Check sheet for the modelled part. Datum: model origin and axes. Units: mm. A direction names the side the tool comes from. Round coordinates to 2 decimals unless told otherwise and drop trailing zeros. Order: outer loops, then holes, each group sorted by start corner. A loop starts at its lowest first (then second) coordinate and runs counter-clockwise, first axis right, second up. Notation, with made-up numbers: M 26.25,49 L 55.25,49 A29 ccw 55.25,74 Z; hole C -34,42 d8. An arc over 180 degrees is marked long. One line per item, written item: value. Start each with the question number.
(1) Cross-section at C-C, the plane y = 4.75. Enter the section's corners in (x, z).
(2) Thickness scan on L1, parallel to Y at x = 1, z = -1.9; L2, parallel to Z at x = -0.1, y = 7.75; L3, parallel to X at y = 0.75, z = 0. Record the ranges inside material, lowest first.
(3) Cross-section at B-B, the plane x = 0. Enter the section's corners in (y, z), and give its area (3 significant figures).
(4) Cross-section at D-D, the plane y = 9. Enter the section's corners in (x, z).
(5) Access from +Z, -Z, +X, -X, +Y, -Y to the whole of each face (thin tool, end or side, straight path). Record for faces 1 (the face through (0, 7, -2)), 2 (the face through (2.685, 8.514, 0.596)).
(6) Depth check by flat-ended pin: pin 1 Ø3 at (x, y) = (-2, 1.5) entering from +Z. Enter the tip coordinate at first touch or a pass-through.
(7) Cross-section at A-A, the plane z = 0. Enter the section's corners in (x, y), and give its area (3 significant figures).
from build123d import *

# Parameters (mm, degrees)
FILLET1_R = 0.5


with BuildPart() as part:
    # Sketch1 → Revolve1 (revolve)
    with BuildSketch(Plane.XY, mode=Mode.PRIVATE) as revolve1_sk:
        Polygon((0, 0), (1.5, 0), (1.5, 7), (2.75, 7), (2.75, 10), (0, 10), (0, 7), align=None)
    revolve(revolve1_sk.sketch.rotate(Axis((0, 0, 0), (0, 1, 0)), 90), axis=Axis((0, 0, 0), (0, 1, 0)))

    # Fillet1
    fillet1_edges = [part.edges().sort_by_distance(p)[0] for p in [
        (0, 7, 2.75),
        (0, 10, 2.75),
    ]]
    fillet(fillet1_edges, radius=FILLET1_R)


solid = part.part
Values found:
1. outline: C 0,0 d3
2. L1: 7 to 10
2. L2: -2.75 to 2.75
2. L3: -1.5 to 1.5
3. outline: M 0,-1.5 L 7,-1.5 L 7,-2.25 A0.5 ccw 7.5,-2.75 L 9.5,-2.75 A0.5 ccw 10,-2.25 L 10,2.25 A0.5 ccw 9.5,2.75 L 7.5,2.75 A0.5 ccw 7,2.25 L 7,1.5 L 0,1.5 Z
3. area: 37.3 mm^2
4. outline: C 0,0 d5.5
5. face 1: -Y
5. face 2: +Y, -Y
6. pin 1: z = 1.41
7. outline: M -2.75,7.5 A0.5 ccw -2.25,7 L -1.5,7 L -1.5,0 L 1.5,0 L 1.5,7 L 2.25,7 A0.5 ccw 2.75,7.5 L 2.75,9.5 A0.5 ccw 2.25,10 L -2.25,10 A0.5 ccw -2.75,9.5 Z
7. area: 37.3 mm^2
